from build123d import *

# Parameters (mm, degrees)
SKETCH1_W           = 25.4
SKETCH1_H           = 25.4
BOSS_EXTRUDE1_DEPTH = 30.6
SKETCH2_W           = 25.4
SKETCH2_H           = 56
BOSS_EXTRUDE2_DEPTH = 3.175


with BuildPart() as part:
    # Sketch1 → Boss-Extrude1 (new body)
    with BuildSketch(Plane(origin=(0, 0, 0), x_dir=(1, 0, 0), z_dir=(0, 1, 0))):
        Rectangle(SKETCH1_W, SKETCH1_H)
    extrude(amount=BOSS_EXTRUDE1_DEPTH)

    # Sketch2 → Boss-Extrude2 (add)
    with BuildSketch(Plane(origin=(12.7, 0, 0), x_dir=(0, 0, -1), z_dir=(1, 0, 0))):
        with Locations((0, 28)):
            Rectangle(SKETCH2_W, SKETCH2_H)
        with BuildLine():
            Line((2.7, 47), (2.7, 37))
            ThreePointArc((2.7, 37), (0, 34.3), (-2.7, 37))
            Line((-2.7, 37), (-2.7, 47))
            ThreePointArc((-2.7, 47), (0, 49.7), (2.7, 47))
        make_face(mode=Mode.SUBTRACT)
    extrude(amount=BOSS_EXTRUDE2_DEPTH)


solid = part.part
The listing builds one solid part. Answer for the finished solid, in the listing's coordinates (mm). A direction names the side the tool comes from. Coordinates: 2 decimals unless noted, no trailing zeros. Order: outer loops, then holes, each group sorted by start corner. A loop starts at its lowest first (then second) coordinate and runs counter-clockwise, first axis right, second up.
Q1. A cutting plane is placed at B-B, the plane y = 42. Write down the section's boundary in (x, z) (3 decimals).
Q2. Which of the six approach directions +Z, -Z, +X, -X, +Y, -Y give full straight-line access (tool end or side, diameter ignored) to faces 1 (the face through (14, 42, 2.7)), 2 (the face through (1, 0, 0)), 3 (the face through (0, 30.6, 0))?
Q3. Given P1, Ø5, axis at x = -6.5, z = 2, coming from the +Y side; P2, Ø12.5, axis at y = 37, z = 4, coming from the -X side, each flat-ended and moving along its own axis, determine where each tip first touches the part or whether it passes through.
Q4. Consider line 1 (Y direction, x = 12.25, z = 2); line 2 (X direction, y = 44.5, z = -5.5) (3 decimals); line 3 (Y direction, x = 14, z = 2). Determine where each line is inside the solid, lowest interval first.
Q5. A cutting plane is placed at A-A, the plane z = 0. Write down the section's boundary in (x, y) (3 decimals).
Q6. A cutting plane is placed at C-C, the plane y = 51. Write down the section's boundary in (x, z) (3 decimals), and give its area (3 significant figures).
Q7. A cutting plane is placed at D-D, the plane x = 7.25. Write down the section's boundary in (y, z), and give its area (3 significant figures).
Q8. For a pull along Z with two mould halves and no side action, classify faces 4 (the face through (14.3, 34.3, -0.1)), 5 (the face through (1, 15, 12.7)), 6 (the face through (-12.7, 15, 0)), 7 (the face through (14.3, 49.7, 0.1)) as pulls with the +Z half, pulls with the -Z half, needs draft (parallel to the pull), parting line crosses it, or undercut.
Answers follow:
1. outline: (12.7, -12.7) - (15.875, -12.7) - (15.875, -2.7) - (12.7, -2.7) - close; (12.7, 2.7) - (15.875, 2.7) - (15.875, 12.7) - (12.7, 12.7) - close
2. face 1: +X, -X
2. face 2: +Z, -Z, +X, -X, -Y
2. face 3: +Z, -Z, -X, +Y
3. P1: stops at y = 30.6
3. P2: stops at x = 12.7
4. line 1: y = 0 to 30.6
4. line 2: x = 12.7 to 15.875
4. line 3: y = 0 to 35.19, 48.81 to 56
5. outline: (-12.7, 0) - (15.875, 0) - (15.875, 34.3) - (12.7, 34.3) - (12.7, 30.6) - (-12.7, 30.6) - close; (12.7, 49.7) - (15.875, 49.7) - (15.875, 56) - (12.7, 56) - close
6. outline: (12.7, -12.7) - (15.875, -12.7) - (15.875, 12.7) - (12.7, 12.7) - close
6. area: 80.6 mm2
7. outline: (0, -12.7) - (30.6, -12.7) - (30.6, 12.7) - (0, 12.7) - close
7. area: 777 mm2
8. face 4: undercut
8. face 5: pulls with the +Z half
8. face 6: needs draft
8. face 7: undercut
